Design review of the part built by this model. Coordinates are the model's own, in mm. Face numbers are marked on the shaded views. A direction names the side the tool comes from. Coordinates: 2 decimals unless noted, no trailing zeros. Loops run counter-clockwise (first coordinate to the right, second up) from the corner with the lowest first, then second, coordinate; pieces in that order, holes last. Notation, with made-up numbers: M -36,-25.75 L -7,-25.75 A25 ccw -7,-1.75 Z; hole C 14.5,10.25 d3. An arc over 180 degrees is marked long. Answer as a JSON object with one key per item and string values. Group by question number.
1. Consider section C-C (z = 0). State the section outline as (x, y) points, then the cut area to 3 significant figures.
2. Insertion check: pin 1 (2.5 mm diameter, centred on y = 4, z = -4, fed in from -X); pin 2 (3 mm diameter, centred on x = -9, z = -1, fed in from +Y); pin 3 (1.7 mm diameter, centred on y = 5, z = -3.5, fed in from +X); pin 4 (3 mm diameter, centred on y = 3, z = -3.5, fed in from -X). Each pin has a flat end and moves straight along its axis. Give the tip position at first contact, or say it passes through.
3. Consider section D-D (y = 5). State the section outline as (x, z) points, then the cut area to 3 significant figures.
4. Consider section B-B (x = -8). State the section outline as (y, z) points.
5. Consider section A-A (y = 3.15). State the section outline as (x, z) points, then the cut area to 3 significant figures.
6. Draft analysis for pull direction Z (two halves, no side actions). For the marked faces 5, 6, 7 and 8, state which applies: +Z half, -Z half, draft (parallel to the pull), parting line (faces both ways), or undercut.
7. Machinability: for the marked faces 1, 2, 3 and 4, which of the approach directions +Z, -Z, +X, -X, +Y, -Y give a long, thin tool a straight path to every point of the face, cutting with its end or side? Answer none if there is none.
8. To check wall thickness, follow probe 1 along X at (y, z) = (0.55, 0); probe 2 along Z at (x, y) = (8, 0.6); probe 3 along X at (y, z) = (0.65, -1). State the ranges of each line that lie inside material, in increasing order.
from build123d import *

# Parameters (mm, degrees)
SKETCH_1_W          = 22
SKETCH_1_H          = 10
EXTRUDE_1_DEPTH     = 6
SKETCH_2_W          = 4
SKETCH_2_H          = 4
CUT_EXTRUDE_1_DEPTH = 24
SKETCH_3_R          = 1.55
CUT_EXTRUDE_2_DEPTH = 6
SKETCH_3_3_R        = 3.05
CUT_EXTRUDE_3_DEPTH = 6


with BuildPart() as part:
    # Sketch 1 → Extrude 1 (new body)
    with BuildSketch(Plane(origin=(0, 0, 0), x_dir=(1, 0, 0), z_dir=(0, 1, 0))):
        Rectangle(SKETCH_1_W, SKETCH_1_H)
    extrude(amount=EXTRUDE_1_DEPTH)

    # Sketch 2 → Cut-Extrude 1 (cut)
    with BuildSketch(Plane.XY.offset(5)):
        with Locations((-9, 4)):
            Rectangle(SKETCH_2_W, SKETCH_2_H)
        with Locations((9, 4)):
            Rectangle(SKETCH_2_W, SKETCH_2_H)
        Polygon((-5, 2), (-5, 0), (5, 0), (5, 2), (5, 4), (-5, 4), align=None)
    extrude(amount=-CUT_EXTRUDE_1_DEPTH, mode=Mode.SUBTRACT)

    # Sketch 3 → Cut-Extrude 2 (cut)
    with BuildSketch(Plane(origin=(0, 2, 0), x_dir=(1, 0, 0), z_dir=(0, 1, 0))):
        with Locations((-8, 0)):
            Circle(SKETCH_3_R)
        with Locations((8, 0)):
            Circle(SKETCH_3_R)
    extrude(amount=-CUT_EXTRUDE_2_DEPTH, mode=Mode.SUBTRACT)

    # Sketch 3_3 → Cut-Extrude 3 (cut)
    with BuildSketch(Plane(origin=(0, 2, 0), x_dir=(1, 0, 0), z_dir=(0, 1, 0))):
        with Locations((-8, 0)):
            Circle(SKETCH_3_3_R)
        with Locations((8, 0)):
            Circle(SKETCH_3_3_R)
    extrude(amount=CUT_EXTRUDE_3_DEPTH, mode=Mode.SUBTRACT)


solid = part.part
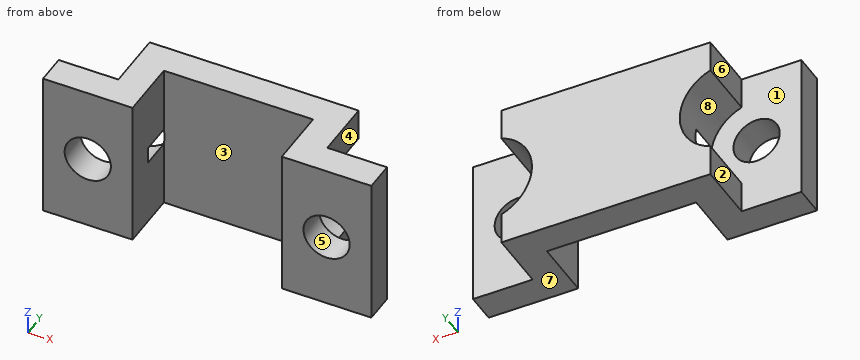
Findings below:
{
 "1": {"outline": "M -11,0 L -9.55,0 L -9.55,2 L -11,2 Z; M -6.45,0 L -5,0 L -5,2 L -6.45,2 Z; M -4.95,4 L 4.95,4 L 4.95,6 L -4.95,6 Z; M 5,0 L 6.45,0 L 6.45,2 L 5,2 Z; M 9.55,0 L 11,0 L 11,2 L 9.55,2 Z", "area": "31.4 mm^2"},
 "2": {"pin 1": "stops at x = -7", "pin 2": "stops at y = 2", "pin 3": "stops at x = 7", "pin 4": "stops at x = -11"},
 "3": {"outline": "M -7,-5 L 7,-5 L 7,-2.88 A3.05 cw 7,2.88 L 7,5 L -7,5 L -7,2.88 A3.05 cw -7,-2.88 Z", "area": "123 mm^2"},
 "4": {"outline": "M 0,-5 L 2,-5 L 2,-1.55 L 0,-1.55 Z; M 0,1.55 L 2,1.55 L 2,5 L 0,5 Z"},
 "5": {"outline": "M -7,-5 L -5,-5 L -5,-0.55 A3.05 cw -7,-2.88 Z; M -7,2.88 A3.05 cw -5,0.55 L -5,5 L -7,5 Z; M 5,-5 L 7,-5 L 7,-2.88 A3.05 cw 5,-0.55 Z; M 5,0.55 A3.05 cw 7,2.88 L 7,5 L 5,5 Z", "area": "22.8 mm^2"},
 "6": {"face 5": "undercut", "face 6": "draft", "face 7": "-Z half", "face 8": "undercut"},
 "7": {"face 1": "-X, +Y", "face 2": "+Z, -Z, -X, +Y", "face 3": "+Z, -Z, -Y", "face 4": "+Z, -Z, +X, +Y"},
 "8": {"probe 1": "x = -11 to -9.55, -6.45 to -5, 5 to 6.45, 9.55 to 11", "probe 2": "z = -5 to -1.55, 1.55 to 5", "probe 3": "x = -11 to -9.18, -6.82 to -5, 5 to 6.82, 9.18 to 11"}
}
